For this review, take the finished solid that the model builds, in its own axes (mm). Face numbers are marked on the shaded views. A direction names the side the tool comes from. Give positions to 0.01 mm unless a question says otherwise; leave off trailing zeros. Write each loop counter-clockwise with the first axis right and the second up, starting at its lowest first coordinate (ties: lowest second). Pieces come first, ordered by that corner, then holes.
Q1. We need section C-C (x = -6). Write out the cut boundary in (y, z).
Q2. We need section B-B (z = 11.5). Write out the cut boundary in (x, y), then the cut area to 3 significant figures.
Q3. Insertion check: P1, Ø14, axis at x = 3, z = -4, coming from the +Y side; P2, Ø5, axis at x = 9.5, z = -6.5, coming from the -Y side; P3, Ø3, axis at x = -23, z = -2.5, coming from the +Y side; P4, Ø3, axis at x = -20, y = 13, coming from the +Z side. Each pin has a flat end and moves straight along its axis. Give the tip position at first contact, or say it passes through.
Q4. Machinability: for the marked faces 4, 5, 6 and 7, which of the approach directions +Z, -Z, +X, -X, +Y, -Y give a long, thin tool a straight path to every point of the face, cutting with its end or side? Answer none if there is none.
Q5. We need section A-A (y = 14). Write out the cut boundary in (x, z).
Q6. Mouldability with a two-part tool opening along X and no side actions: class the marked faces 1, 2 and 3 as released by +X, released by -X, zero draft, split by the parting line, or undercut.
Q7. We need section D-D (y = 8.25). Write out the cut boundary in (x, z), then the cut area to 3 significant figures.
Q8. For line 1 (X direction, y = 14, z = -2.5); line 2 (Y direction, x = -5, z = -2.5); line 3 (Y direction, x = 21.5, z = 1), list the stretches that pass through material, from the lowest coordinate up.
```python
from build123d import *

# Parameters (mm, degrees)
SKETCH1_W           = 58
SKETCH1_H           = 34
BOSS_EXTRUDE1_DEPTH = 10
SKETCH3_W           = 23
SKETCH3_H           = 7
CUT_EXTRUDE1_DEPTH  = 34
SKETCH4_W           = 11.75
SKETCH4_H           = 7
CUT_EXTRUDE2_DEPTH  = 34
SKETCH6_W           = 3
SKETCH6_H           = 34
BOSS_EXTRUDE2_DEPTH = 13
FILLET1_R           = 1


with BuildPart() as part:
    # Sketch1 → Boss-Extrude1 (new body)
    with BuildSketch(Plane(origin=(0, 0, 0), x_dir=(1, 0, 0), z_dir=(0, 1, 0))):
        Rectangle(SKETCH1_W, SKETCH1_H)
    extrude(amount=BOSS_EXTRUDE1_DEPTH)

    # Sketch3 → Cut-Extrude1 (cut)
    with BuildSketch(Plane.XY.offset(17)):
        with Locations((0, 3.5)):
            Rectangle(SKETCH3_W, SKETCH3_H)
    extrude(amount=-CUT_EXTRUDE1_DEPTH, mode=Mode.SUBTRACT)

    # Sketch4 → Cut-Extrude2 (cut)
    with BuildSketch(Plane.XY.offset(17)):
        with Locations((23.125, 6.5)):
            Rectangle(SKETCH4_W, SKETCH4_H)
    cut_extrude2 = extrude(amount=-CUT_EXTRUDE2_DEPTH, mode=Mode.SUBTRACT)

    # Mirror1: Cut-Extrude2 across plane
    add(cut_extrude2.mirror(Plane(origin=(0, 0, 0), x_dir=(0, 0, 1), z_dir=(1, 0, 0))), mode=Mode.SUBTRACT)

    # Sketch6 → Boss-Extrude2 (add)
    with BuildSketch(Plane(origin=(0, 10, 0), x_dir=(1, 0, 0), z_dir=(0, 1, 0))):
        with Locations((15.75, 0)):
            Rectangle(SKETCH6_W, SKETCH6_H)
    boss_extrude2 = extrude(amount=BOSS_EXTRUDE2_DEPTH)

    # Mirror2: Boss-Extrude2 across plane
    add(boss_extrude2.mirror(Plane(origin=(0, 0, 0), x_dir=(0, 0, 1), z_dir=(1, 0, 0))))

    # Fillet1
    fillet1_edges = [part.edges().sort_by_distance(p)[0] for p in [
        (-11.5, 0, 0),
        (-11.5, 7, 0),
        (11.5, 7, 0),
        (11.5, 0, 0),
        (17.25, 3, 0),
        (-17.25, 3, 0),
    ]]
    fillet(fillet1_edges, radius=FILLET1_R)


solid = part.part
```
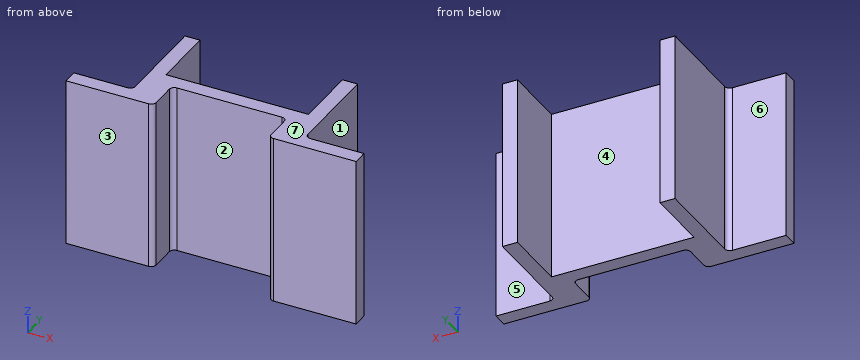
Computed:
1. outline: (7, -17) - (10, -17) - (10, 17) - (7, 17) - close
2. outline: (-29, 0) - (-12.5, 0) arc R1 ccw to (-11.5, 1) - (-11.5, 6) arc R1 cw to (-10.5, 7) - (10.5, 7) arc R1 cw to (11.5, 6) - (11.5, 1) arc R1 ccw to (12.5, 0) - (29, 0) - (29, 3) - (18.25, 3) arc R1 cw to (17.25, 4) - (17.25, 23) - (14.25, 23) - (14.25, 10) - (-14.25, 10) - (-14.25, 23) - (-17.25, 23) - (-17.25, 4) arc R1 cw to (-18.25, 3) - (-29, 3) - close
2. area: 333 mm2
3. P1: stops at y = 10
3. P2: stops at y = 0.13
3. P3: stops at y = 3
3. P4: passes through
4. face 4: +Z, -Z, +Y
4. face 5: +Z, -Z, +X, +Y
4. face 6: +Z, -Z, -X, +Y
4. face 7: +Z, +X, -X, +Y, -Y
5. outline: (-17.25, -17) - (-14.25, -17) - (-14.25, 17) - (-17.25, 17) - close; (14.25, -17) - (17.25, -17) - (17.25, 17) - (14.25, 17) - close
6. face 1: released by +X
6. face 2: undercut
6. face 3: zero draft
7. outline: (-17.25, -17) - (17.25, -17) - (17.25, 17) - (-17.25, 17) - close
7. area: 1,170 mm2
8. line 1: x = -17.25 to -14.25, 14.25 to 17.25
8. line 2: y = 7 to 10
8. line 3: y = 0 to 3
